Build history of the part. All positions in model axes, mm. A direction names the side the tool comes from. Give positions to 0.01 mm unless a question says otherwise; leave off trailing zeros.
1) 3-axis set-ups, long thin cutter, end or side, ignore diameter. For faces 4 (the flat face through (650, 75, 17)), 5 (the flat face through (776.72, -28.3, -32.3)), 6 (the flat face through (610, -43, -43)), 7 (the cylindrical face through (219.7, -12.6, 30.5)), 8 (the cylindrical face through (624.65, 47.681, 62.184)): which of +Z, -Z, +X, -X, +Y, -Y reach the whole face in a straight line?
2) Band-saw the part on A-A on x = 615.5. State how many separate pieces and enclosed holes the cut face has, then the cut area to 3 significant figures.
3) Wall check: line 1 (Y direction, x = 674.75, z = 0); line 2 (Y direction, x = 302, z = 0); line 3 (Y direction, x = 322.5, z = 0). Give the ranges that are in metal, low to high.
4) Two-plate mould, pull along Y, no slides. Class faces 1 (the cylindrical face through (682.21, -69.376, -3.576)), 2 (the cylindrical face through (736.3, 36.71, 39.6)), 3 (the flat face through (697, 50, 22)): +Y half, -Y half, draft (parallel to the pull), parting line (faces both ways), or undercut.
5) Flat gauge pins, fed straight in: P1, Ø3.5, axis at y = 20, z = 0, coming from the +X side; P2, Ø6, axis at y = 59, z = -47.5, coming from the +X side; P3, Ø2, axis at x = 604, z = 42, coming from the -Y side; P4, Ø1.5, axis at y = 12, z = 18.5, coming from the -X side. Where does each tip first touch, or does it go through?
```python
from build123d import *

# Parameters (mm, degrees)
CUT_EXTRUDE1_DEPTH = 400
SKETCH3_R          = 33
SKETCH3_R_2        = 3.1000000000000028
CUT_EXTRUDE2_DEPTH = 40
SKETCH3_2_R        = 3.1000000000000028
CUT_EXTRUDE4_DEPTH = 588.2704126987336
SKETCH4_R          = 7.750000000000002
SKETCH4_R_2        = 7.749999999999998
SKETCH4_R_3        = 7.75
CUT_EXTRUDE5_DEPTH = 30
CUT_EXTRUDE6_START = -166.72
CUT_EXTRUDE6_DEPTH = 166.72
CUT_EXTRUDE7_START = -166.72
CUT_EXTRUDE7_DEPTH = 40
FILLET1_R          = 3
FILLET2_R          = 1


# Read off the part's stored shape, not the designer's step: Cut-Extrude7
with BuildPart() as part:
    # Sketch1 → Revolve1 (revolve)
    with BuildSketch(Plane.XY, mode=Mode.PRIVATE) as revolve1_sk:
        with BuildLine():
            Line((650.0000000000001, 78.36), (600.0000000000001, 78.35999999999999))
            add(Edge.make_bspline(
                [(200.00000000000358, 42.32828037010144), (208.17052038042252, 43.51395402277683), (225.68488706430128, 45.99527814756255), (252.5646252490451, 49.61720291886234), (288.8377795121088, 54.154525537406215), (326.32073414086074, 58.489281573967666), (363.84117713275197, 62.4863121261995), (401.3959942076804, 66.1465092198773), (438.98297125108434, 69.46060873551288), (476.60065297069735, 72.40710938265987), (509.54226569024473, 74.62869781075653), (537.7964811389767, 76.23350465282824), (560.2922621801154, 77.27545940077594), (575.1953567037801, 77.83264328043563), (587.2142250450652, 78.17300672656529), (594.5199761893905, 78.31035588184413), (598.173256760109, 78.35432466011183), (600.0000000000001, 78.35999999999999)],
                knots=[0.33782774337518406, 0.33782774337518406, 0.33782774337518406, 0.33782774337518406, 0.33782774337518406, 0.3922467059008778, 0.45442341660838875, 0.5166001272068571, 0.5787768404127641, 0.6409535517353824, 0.7031302632972144, 0.7653069754242735, 0.8274836869805778, 0.8896603985814769, 0.9207487548355946, 0.9518371110897123, 0.9759185555448562, 0.9879592777724281, 1, 1, 1, 1, 1], degree=4))
            Line((200.0000000000036, 42.32828037010143), (200, -7.43e-14))
            Line((200, 0), (776.72, 0))
            Line((776.72, 0), (776.72, 54))
            Line((776.72, 54), (697.0000000000002, 54))
            Line((697.0000000000002, 54), (697.0000000000002, 76.20000000000005))
            Line((697.0000000000002, 76.20000000000005), (650.0000000000001, 76.20000000000005))
            Line((650.0000000000001, 76.20000000000005), (650.0000000000001, 78.36))
        make_face()
    revolve(revolve1_sk.sketch.rotate(Axis((776.72, 0, 0), (-1, 0, 0)), 90), axis=Axis((776.72, 0, 0), (-1, 0, 0)))

    # Sketch2 → Cut-Extrude1 (cut)
    with BuildSketch(Plane(origin=(776.72, 0, 0), x_dir=(0, 0, -1), z_dir=(1, 0, 0))):
        with BuildLine():
            ThreePointArc((47.36738574096539, -16.010333165383813), (-35.35533905932756, 35.35533905932719), (16.01033316538431, -47.367385740965226))
            ThreePointArc((16.010333165384957, -47.36738574096489), (14.843408327061695, -43.77194076139418), (14.25549204864172, -40.03786890496388))
            ThreePointArc((14.25549204864269, -40.03786890496403), (30.05203820042843, -30.05203820042811), (40.037868904964185, -14.255492048642266))
            ThreePointArc((40.03786890496402, -14.255492048641287), (43.77194076139434, -14.843408327061226), (47.36738574096508, -16.01033316538445))
        make_face()
    extrude(amount=-CUT_EXTRUDE1_DEPTH, mode=Mode.SUBTRACT)

    # Sketch3 → Cut-Extrude2 (cut)
    with BuildSketch(Plane.ZY.offset(-200.00000000000273)):
        Circle(SKETCH3_R)
        with Locations((0, 20)):
            Circle(SKETCH3_R_2, mode=Mode.SUBTRACT)
        with Locations((0, -20)):
            Circle(SKETCH3_R_2, mode=Mode.SUBTRACT)
    extrude(amount=-CUT_EXTRUDE2_DEPTH, mode=Mode.SUBTRACT)

    # Sketch3<2> → Cut-Extrude4 (cut, through all)
    with BuildSketch(Plane.ZY.offset(-200.00000000000273)):
        with Locations((0, 20)):
            Circle(SKETCH3_2_R)
        with Locations((0, -20)):
            Circle(SKETCH3_2_R)
    extrude(amount=-CUT_EXTRUDE4_DEPTH, mode=Mode.SUBTRACT)

    # Sketch4 → Cut-Extrude5 (cut)
    with BuildSketch(Plane(origin=(697.0000000000002, 0, 0), x_dir=(0, 0, -1), z_dir=(1, 0, 0))):
        with Locations((0, 62.5)):
            Circle(SKETCH4_R)
        with Locations((62.499999999999986, -2.1825e-13)):
            Circle(SKETCH4_R_2)
        with Locations((-4.3715e-13, -62.5)):
            Circle(SKETCH4_R_3)
        with Locations((-62.49999999999999, 6.5573e-13)):
            Circle(SKETCH4_R_2)
    extrude(amount=-CUT_EXTRUDE5_DEPTH, mode=Mode.SUBTRACT)

    # Sketch2<3> → Cut-Extrude6 (cut)
    with BuildSketch(Plane(origin=(776.72, 0, 0), x_dir=(0, 0, -1), z_dir=(1, 0, 0)).offset(CUT_EXTRUDE6_START)):
        with BuildLine():
            ThreePointArc((18.674162122276517, -42.585510083018875), (19.845504593214095, -46.16550545726443), (21.667324002424465, -49.462380356933224))
            ThreePointArc((21.66732400242451, -49.46238035693348), (38.18376618407376, -38.18376618407337), (49.4623803569337, -21.667324002424003))
            ThreePointArc((49.46238035693346, -21.667324002423932), (46.16550545726464, -19.845504593213597), (42.58551008301907, -18.67416212227606))
            ThreePointArc((42.58551008301935, -18.674162122276265), (32.880465325174626, -32.88046532517429), (18.674162122276698, -42.58551008301916))
        make_face()
    extrude(amount=CUT_EXTRUDE6_DEPTH, mode=Mode.SUBTRACT)

    # Cut-Extrude7 outline → Cut-Extrude7 (cut)
    with BuildSketch(Plane(origin=(776.72, 0, 0), x_dir=(0, 0, -1), z_dir=(1, 0, 0)).offset(CUT_EXTRUDE7_START)):
        with BuildLine():
            ThreePointArc((49.462380357, -21.667324002), (38.183766184, -38.183766184), (21.667324002, -49.462380357))
            ThreePointArc((21.667324002, -49.462380357), (52.325901808, -52.325901808), (49.462380357, -21.667324002))
        make_face()
    extrude(amount=CUT_EXTRUDE7_DEPTH, mode=Mode.SUBTRACT)

    # Fillet1
    # the kernel refuses this fillet: 3 mm, written as the material it takes off along each edge
    with BuildSketch(Plane(origin=(783.0040750376627, -40.03786890496436, -14.255492048641756), x_dir=(0, 0.36048933664361255, -0.9327633344885766), z_dir=(-1, 0, 0))) as fillet1_piece_1:
        with BuildLine():
            CenterArc((2.3526530908588352, 2.998927692547355), FILLET1_R, 190.6958961912189, 77.77213613267259)
            ThreePointArc((-0.5952251863106816, 2.4421389866704493), (-0.3296065941102598, 1.2132715607510574), (0, 0))
            ThreePointArc((0, 0), (1.1362245041079626, 0.01519102224578455), (2.2724490082159248, 3e-17))
        make_face()
    extrude(amount=406.28407503766266, mode=Mode.SUBTRACT)
    with BuildSketch(Plane(origin=(783.0040750376628, -14.255492048641326, -40.03786890496452), x_dir=(0, -0.12935906708338796, -0.9915978175466682), z_dir=(-1, 0, 0))) as fillet1_piece_2:
        with BuildLine():
            CenterArc((2.356528139123201, 2.995883676075499), FILLET1_R, 195.22966173823434, 77.77213613267247)
            ThreePointArc((-0.5381137542877349, 2.207817492997983), (-0.25429790806270375, 1.1075059660548925), (0, 0))
            ThreePointArc((0, 0), (1.2568150075323716, -0.0329305913960081), (2.513630015064742, 0))
        make_face()
    extrude(amount=406.2840750376628, mode=Mode.SUBTRACT)
    with BuildSketch(Plane(origin=(697.0000000000002, -49.46238035693335, -21.667324002424486), x_dir=(0, -0.3710376913926641, 0.9286178070476584), z_dir=(1, 0, 0))) as fillet1_piece_3:
        with BuildLine():
            CenterArc((3.4382745469761065, -2.998391169718282), FILLET1_R, 88.12348720794618, 95.23374468145443)
            ThreePointArc((0.4434230907932443, -3.1740748496643687), (0.2853925875390597, -1.5781410862550613), (0, 0))
            ThreePointArc((0, 0), (1.7682554813020526, 0.0289589450709421), (3.5365109626041082, -1.1e-16))
        make_face()
    extrude(amount=88.56127740651004, mode=Mode.SUBTRACT)
    with BuildSketch(Plane(origin=(697.0000000000002, -21.667324002423964, -49.46238035693357), x_dir=(0, 0.9286178070476617, -0.3710376913926558), z_dir=(1, 0, 0))) as fillet1_piece_4:
        with BuildLine():
            CenterArc((3.438274546976126, 2.998391169718279), FILLET1_R, 176.64276811059946, 95.23374468145443)
            ThreePointArc((0.44342309079326614, 3.174074849664362), (0.28539258753907326, 1.5781410862550511), (0, 0))
            ThreePointArc((0, 0), (1.7682554813020637, -0.02895894507093817), (3.53651096260413, 5e-17))
        make_face()
    extrude(amount=88.56127740651004, mode=Mode.SUBTRACT)

    # Fillet2
    fillet2_edges = [part.edges().sort_by_distance(p)[0] for p in [
        (576.72, -47.36738574096506, -16.010333165384637),
        (576.72, -16.01033316538413, -47.36738574096523),
        (693.36, -18.67416212227616, -42.58551008301921),
        (693.36, -42.58551008301902, -18.674162122276606),
    ]]
    fillet(fillet2_edges, radius=FILLET2_R)


solid = part.part
```
Findings below:
1. face 4: +X
1. face 5: +Z, -Z, +X, +Y, -Y
1. face 6: none
1. face 7: -X
1. face 8: +X, -X
2. separate pieces: 1
2. enclosed holes: 2
2. area: 10,800 mm2
3. line 1: y = -76.2 to -70.25, -54.75 to -50, 50 to 54.75, 70.25 to 76.2
3. line 2: y = -55.64 to -23.1, -16.9 to 16.9, 23.1 to 55.64
3. line 3: y = -57.99 to -23.1, -16.9 to 16.9, 23.1 to 57.99
4. face 1: undercut
4. face 2: parting line
4. face 3: draft
5. P1: passes through
5. P2: stops at x = 697
5. P3: stops at y = -66.78
5. P4: stops at x = 240
